Print and shaded views of the part. All mm, measured from the part's lowest x, y and z. A direction names the side the tool comes from. Give positions to 0.01 mm unless a question says otherwise; leave off trailing zeros. Order: outer loops, then holes, each group sorted by start corner. A loop starts at its lowest first (then second) coordinate and runs counter-clockwise, first axis right, second up. Notation, with made-up numbers: (86, 78.5) - (104, 78.5) arc R24 cw to (104, 92.5) - close; hole circle Ø1 at (59, -25). An arc over 180 degrees is marked (long way). Answer in a Markdown table with one row per item.
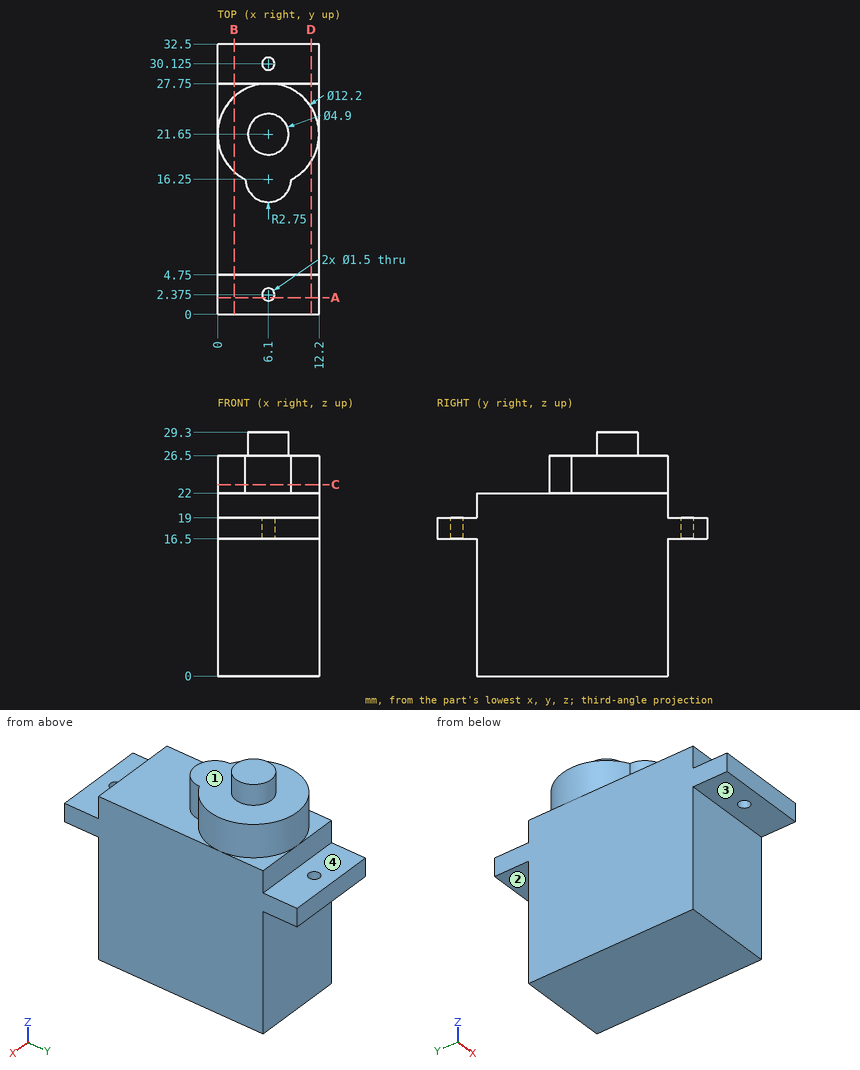
1. Cut at A-A on y = 2. Write the cut outline in (x, z), and give its area (3 significant figures).
Check result:
| item | result |
|---|---|
| outline | (0, 16.5) - (5.45, 16.5) - (5.45, 19) - (0, 19) - close; (6.75, 16.5) - (12.2, 16.5) - (12.2, 19) - (6.75, 19) - close |
| area | 27.3 mm² |
2. Cut at D-D on x = 11.25. Write the cut outline in (y, z), and give its area (3 significant figures).
Check result:
| item | result |
|---|---|
| outline | (0, 16.5) - (4.75, 16.5) - (4.75, 0) - (27.75, 0) - (27.75, 16.5) - (32.5, 16.5) - (32.5, 19) - (27.75, 19) - (27.75, 22) - (24.92, 22) - (24.92, 26.5) - (18.38, 26.5) - (18.38, 22) - (4.75, 22) - (4.75, 19) - (0, 19) - close |
| area | 559 mm² |
3. Drop flat-ended pins along their axis: P1, Ø1.5, axis at x = 10, y = 14.5, coming from the -Z side; P2, Ø1.5, axis at x = 7, z = 20, coming from the -Y side; P3, Ø1.5, axis at x = 3, z = 9.5, coming from the +Y side; P4, Ø5, axis at x = 7.5, y = 1.5, coming from the -Z side. Give the stop position or say it passes through.
Check result:
| item | result |
|---|---|
| P1 | stops at z = 0 |
| P2 | stops at y = 4.75 |
| P3 | stops at y = 27.75 |
| P4 | stops at z = 16.5 |
4. Cut at B-B on x = 2. Write the cut outline in (y, z), and give its area (3 significant figures).
Check result:
| item | result |
|---|---|
| outline | (0, 16.5) - (4.75, 16.5) - (4.75, 0) - (27.75, 0) - (27.75, 16.5) - (32.5, 16.5) - (32.5, 19) - (27.75, 19) - (27.75, 22) - (26.17, 22) - (26.17, 26.5) - (17.13, 26.5) - (17.13, 22) - (4.75, 22) - (4.75, 19) - (0, 19) - close |
| area | 570 mm² |
5. Probe line 1 (Y direction, x = 6.1, z = 17.65) (3 decimals); line 2 (Z direction, x = 10, y = 25); line 3 (Y direction, x = 1.25, z = 21). List the from-to ranges inside material, lowest first.
Check result:
| item | result |
|---|---|
| line 1 | y = 0 to 1.625, 3.125 to 29.375, 30.875 to 32.5 |
| line 2 | z = 0 to 26.5 |
| line 3 | y = 4.75 to 27.75 |
6. Cut at C-C on z = 23. Write the cut outline in (x, y), and give its area (3 significant figures).
Check result:
| item | result |
|---|---|
| outline | (3.35, 16.2) arc R2.75 ccw to (8.85, 16.2) arc R6.1 ccw (long way) to start |
| area | 126 mm² |
7. Which spindle directions (+Z, -Z, +X, -X, +Y, -Y) get a long thin tool onto all of the face, cutting with end or side? Do the marked faces 1, 2, 3 and 4. Say none if no direction does.
Check result:
| item | result |
|---|---|
| face 1 | +Z |
| face 2 | -Z, +X, -X, +Y |
| face 3 | -Z, +X, -X, -Y |
| face 4 | +Z, +X, -X, +Y |
